Check sheet for the modelled part. Datum: model origin and axes. Units: mm. A direction names the side the tool comes from. Round coordinates to 2 decimals unless told otherwise and drop trailing zeros. Order: outer loops, then holes, each group sorted by start corner. A loop starts at its lowest first (then second) coordinate and runs counter-clockwise, first axis right, second up.
(1) Thickness scan on probe 1 along X at (y, z) = (0, -2.5); probe 2 along X at (y, z) = (0, -2.35); probe 3 along Z at (x, y) = (6, 9). Record the ranges inside material, lowest first.
(2) Tool access check on faces 1 (the flat face through (30, -30, 8)), 2 (the cylindrical face through (-8.498, 38.268, -2.26)), 3 (the cylindrical face through (37.745, 26.292, 1.958)), 4 (the cylindrical face through (33.643, -23.434, 9.86)), 5 (the conical face through (36.731, 25.586, -2.236)). Record the directions out of +Z, -Z, +X, -X, +Y, -Y that give a thin tool (end or side, any length) a straight path to the whole face; none if there is none.
(3) Sectioned sample at B-B, the plane z = 17. Count the separate pieces of the cut face and the enclosed holes in it, and give its area (3 significant figures).
(4) Sectioned sample at A-A, the plane z = 3.75. Enter the section's corners in (x, y), and give its area (3 significant figures).
(5) Mould release check, pull along X, two halves, no side actions. Record for faces 6 (the conical face through (34.102, 23.754, 19.441)), 7 (the flat face through (-36, 20, -3)), 8 (the flat face through (-30, 30, 8)): released by +X, released by -X, zero draft, split by the parting line, or undercut.
(6) Depth check by flat-ended pin: pin 1 (1 mm diameter, centred on x = -32.5, z = 8, fed in from +Y); pin 2 (1.5 mm diameter, centred on x = -15, y = -9.5, fed in from +Z); pin 3 (5 mm diameter, centred on y = 17, z = 16.5, fed in from +X). Enter the tip coordinate at first touch or a pass-through.
```python
from build123d import *
from build123d import SkipClean  # not in build123d's __all__

# Parameters (mm, degrees)
F1_DEPTH    = 20
F2_SIZE     = 4.99999
F2_2_SIZE   = 4.99999
F2_3_SIZE   = 4.99999
F2_4_SIZE   = 4.99999
F3_DEPTH    = 3
F4_SIZE     = 5
F5_R        = 41
F5_R_2      = 39.2
F6_DEPTH    = 1.5
F7_SIZE     = 5
F8_T2_ANGLE = 50
F8_T4_ANGLE = 90
F8_T6_ANGLE = 50
F8_T8_ANGLE = 90
F9_SIZE     = 2


# Not quite as in the source:
# - a fillet or chamfer that OpenCascade refuses, or shapes differently, is made with other operations: its cross-section is extruded or revolved along the edge and cut away or added
# - a fillet or chamfer is up to 0.001 mm smaller than in the source, because OpenCascade refuses the exact size


with BuildPart() as f1:
    # F0 (on Top) → F1 (new body)
    with BuildSketch(Plane.XY):
        with BuildLine():
            ThreePointArc((-37.1586192685, 17.3273487314), (-33.5852338158, 23.5166338904), (-28.9913780286, 28.9913780286))
            Line((-28.9913780286, 28.9913780286), (-32.5269119346, 32.5269119346))
            ThreePointArc((-32.5269119346, 32.5269119346), (-37.6809940373, 26.3845160721), (-41.6901582037, 19.4404400401))
            Line((-41.6901582037, 19.4404400401), (-37.1586192685, 17.3273487314))
        make_face()
    extrude(amount=F1_DEPTH)

    # F2 (size 5 in the source; OpenCascade refuses exactly that, so slightly less here)
    f2_edges = [f1.edges().sort_by_distance(p)[0] for p in [
        (-37.680994, 26.384516, 20),
    ]]
    chamfer(f2_edges, length=F2_SIZE)



with BuildPart() as f1b:
    # F0 (on Top) → F1, piece 2 (new body)
    with BuildSketch(Plane.XY):
        with BuildLine():
            ThreePointArc((28.9913780286, 28.9913780286), (33.5852338158, 23.5166338904), (37.1586192685, 17.3273487314))
            Line((37.1586192685, 17.3273487314), (41.6901582037, 19.4404400401))
            ThreePointArc((41.6901582037, 19.4404400401), (37.6809940373, 26.3845160721), (32.5269119346, 32.5269119346))
            Line((32.5269119346, 32.5269119346), (28.9913780286, 28.9913780286))
        make_face()
    extrude(amount=F1_DEPTH)

    # F2#2 (size 5 in the source; OpenCascade refuses exactly that, so slightly less here)
    f2_2_edges = [f1b.edges().sort_by_distance(p)[0] for p in [
        (37.680994, 26.384516, 20),
    ]]
    chamfer(f2_2_edges, length=F2_2_SIZE)


with BuildPart() as f1c:
    # F0 (on Top) → F1, piece 3 (new body)
    with BuildSketch(Plane.XY):
        with BuildLine():
            Line((-32.5269119346, -32.5269119346), (-28.9913780286, -28.9913780286))
            ThreePointArc((-28.9913780286, -28.9913780286), (-33.5852338158, -23.5166338904), (-37.1586192685, -17.3273487314))
            Line((-37.1586192685, -17.3273487314), (-41.6901582037, -19.4404400401))
            ThreePointArc((-41.6901582037, -19.4404400401), (-37.6809940373, -26.3845160721), (-32.5269119346, -32.5269119346))
        make_face()
    extrude(amount=F1_DEPTH)

    # F2#3 (size 5 in the source; OpenCascade refuses exactly that, so slightly less here)
    f2_3_edges = [f1c.edges().sort_by_distance(p)[0] for p in [
        (-37.680994, -26.384516, 20),
    ]]
    chamfer(f2_3_edges, length=F2_3_SIZE)


with BuildPart() as f1d:
    # F0 (on Top) → F1, piece 4 (new body)
    with BuildSketch(Plane.XY):
        with BuildLine():
            Line((41.6901582037, -19.4404400401), (37.1586192685, -17.3273487314))
            ThreePointArc((37.1586192685, -17.3273487314), (33.5852338158, -23.5166338904), (28.9913780286, -28.9913780286))
            Line((28.9913780286, -28.9913780286), (32.5269119346, -32.5269119346))
            ThreePointArc((32.5269119346, -32.5269119346), (37.6809940373, -26.3845160721), (41.6901582037, -19.4404400401))
        make_face()
    extrude(amount=F1_DEPTH)

    # F2#4 (size 5 in the source; OpenCascade refuses exactly that, so slightly less here)
    f2_4_edges = [f1d.edges().sort_by_distance(p)[0] for p in [
        (37.680994, -26.384516, 20),
    ]]
    chamfer(f2_4_edges, length=F2_4_SIZE)


with BuildPart() as f1_1:
    add(f1.part, clean=False)

    with SkipClean():  # cleaning this boolean's faces spoils the solid; the shape is the same uncleaned
        add(f1b.part)  # F3 merges F1b

    with SkipClean():  # cleaning this boolean's faces spoils the solid; the shape is the same uncleaned
        add(f1c.part)  # F3 merges F1c

    with SkipClean():  # cleaning this boolean's faces spoils the solid; the shape is the same uncleaned
        add(f1d.part)  # F3 merges F1d
    # F0 (on Top) → F3 (join)
    with BuildSketch(Plane.XY):
        with BuildLine():
            ThreePointArc((-37.1586192685, 17.3273487314), (-33.5852338158, 23.5166338904), (-28.9913780286, 28.9913780286))
            Line((-28.9913780286, 28.9913780286), (-32.5269119346, 32.5269119346))
            ThreePointArc((-32.5269119346, 32.5269119346), (-37.6809940373, 26.3845160721), (-41.6901582037, 19.4404400401))
            Line((-41.6901582037, 19.4404400401), (-37.1586192685, 17.3273487314))
        make_face()
        with BuildLine():
            Line((32.5269119346, -32.5269119346), (28.9913780286, -28.9913780286))
            ThreePointArc((28.9913780286, -28.9913780286), (0, -41), (-28.9913780286, -28.9913780286))
            Line((-28.9913780286, -28.9913780286), (-32.5269119346, -32.5269119346))
            ThreePointArc((-32.5269119346, -32.5269119346), (0, -46), (32.5269119346, -32.5269119346))
        make_face()
        with BuildLine():
            ThreePointArc((28.9913780286, 28.9913780286), (33.5852338158, 23.5166338904), (37.1586192685, 17.3273487314))
            Line((37.1586192685, 17.3273487314), (41.6901582037, 19.4404400401))
            ThreePointArc((41.6901582037, 19.4404400401), (37.6809940373, 26.3845160721), (32.5269119346, 32.5269119346))
            Line((32.5269119346, 32.5269119346), (28.9913780286, 28.9913780286))
        make_face()
        with BuildLine():
            ThreePointArc((-28.9913780286, 28.9913780286), (0, 41), (28.9913780286, 28.9913780286))
            Line((28.9913780286, 28.9913780286), (32.5269119346, 32.5269119346))
            ThreePointArc((32.5269119346, 32.5269119346), (0, 46), (-32.5269119346, 32.5269119346))
            Line((-32.5269119346, 32.5269119346), (-28.9913780286, 28.9913780286))
        make_face()
        with BuildLine():
            ThreePointArc((37.1586192685, -17.3273487314), (40.0281362919, -8.8740241715), (41, 0))
            ThreePointArc((41, 0), (40.0281362919, 8.8740241715), (37.1586192685, 17.3273487314))
            ThreePointArc((37.1586192685, 17.3273487314), (33.5852338158, 23.5166338904), (28.9913780286, 28.9913780286))
            ThreePointArc((28.9913780286, 28.9913780286), (0, 41), (-28.9913780286, 28.9913780286))
            ThreePointArc((-28.9913780286, 28.9913780286), (-33.5852338158, 23.5166338904), (-37.1586192685, 17.3273487314))
            ThreePointArc((-37.1586192685, 17.3273487314), (-41, 0), (-37.1586192685, -17.3273487314))
            ThreePointArc((-37.1586192685, -17.3273487314), (-33.5852338158, -23.5166338904), (-28.9913780286, -28.9913780286))
            ThreePointArc((-28.9913780286, -28.9913780286), (0, -41), (28.9913780286, -28.9913780286))
            ThreePointArc((28.9913780286, -28.9913780286), (33.5852338158, -23.5166338904), (37.1586192685, -17.3273487314))
        make_face()
        with BuildLine():
            Line((-32.5269119346, -32.5269119346), (-28.9913780286, -28.9913780286))
            ThreePointArc((-28.9913780286, -28.9913780286), (-33.5852338158, -23.5166338904), (-37.1586192685, -17.3273487314))
            Line((-37.1586192685, -17.3273487314), (-41.6901582037, -19.4404400401))
            ThreePointArc((-41.6901582037, -19.4404400401), (-37.6809940373, -26.3845160721), (-32.5269119346, -32.5269119346))
        make_face()
        with BuildLine():
            Line((41.6901582037, -19.4404400401), (37.1586192685, -17.3273487314))
            ThreePointArc((37.1586192685, -17.3273487314), (33.5852338158, -23.5166338904), (28.9913780286, -28.9913780286))
            Line((28.9913780286, -28.9913780286), (32.5269119346, -32.5269119346))
            ThreePointArc((32.5269119346, -32.5269119346), (37.6809940373, -26.3845160721), (41.6901582037, -19.4404400401))
        make_face()
        with BuildLine():
            ThreePointArc((37.1586192685, 17.3273487314), (40.0281362919, 8.8740241715), (41, 0))
            ThreePointArc((41, 0), (40.0281362919, -8.8740241715), (37.1586192685, -17.3273487314))
            Line((37.1586192685, -17.3273487314), (41.6901582037, -19.4404400401))
            ThreePointArc((41.6901582037, -19.4404400401), (44.9096163275, -9.9562222412), (46, 0))
            ThreePointArc((46, 0), (44.9096163275, 9.9562222412), (41.6901582037, 19.4404400401))
            Line((41.6901582037, 19.4404400401), (37.1586192685, 17.3273487314))
        make_face()
        with BuildLine():
            ThreePointArc((-37.1586192685, -17.3273487314), (-41, 0), (-37.1586192685, 17.3273487314))
            Line((-37.1586192685, 17.3273487314), (-41.6901582037, 19.4404400401))
            ThreePointArc((-41.6901582037, 19.4404400401), (-46, 0), (-41.6901582037, -19.4404400401))
            Line((-41.6901582037, -19.4404400401), (-37.1586192685, -17.3273487314))
        make_face()
    with SkipClean():  # cleaning this boolean's faces spoils the solid; the shape is the same uncleaned
        extrude(amount=-F3_DEPTH)

    # F4
    f4_edges = [f1_1.edges().sort_by_distance(p)[0] for p in [
        (-37.680994, -26.384516, 15.00001),
        (-37.680994, 26.384516, 15.00001),
        (37.680994, -26.384516, 15.00001),
        (37.680994, 26.384516, 15.00001),
    ]]
    chamfer(f4_edges, length=F4_SIZE)

    # F5 (on face) → F6 (cut)
    with BuildSketch(Plane(origin=(0, 0, -3), x_dir=(1, 0, 0), z_dir=(0, 0, -1))):
        Circle(F5_R)
        Circle(F5_R_2, mode=Mode.SUBTRACT)
    with SkipClean():  # cleaning this boolean's faces spoils the solid; the shape is the same uncleaned
        extrude(amount=-F6_DEPTH, mode=Mode.SUBTRACT)

    # F7
    f7_edges = [f1_1.edges().sort_by_distance(p)[0] for p in [
        (-37.680994, -26.384516, 10.00001),
        (37.680994, -26.384516, 10.00001),
        (37.680994, 26.384516, 10.00001),
        (-37.680994, 26.384516, 10.00001),
    ]]
    chamfer(f7_edges, length=F7_SIZE)

    # F8: chamfer of 5 on 4 edges, made by hand

    # F8_s1 → F8_t2 (revolve, cut)
    with BuildSketch(Plane(origin=(0, 0, 0), x_dir=(0, 0, 1), z_dir=(0.4226182617, 0.906307787, 0))):
        Polygon((0, -41), (-5, -46), (0, -46), align=None)
    revolve(axis=Axis((0, 0, 0), (0, 0, 1)), revolution_arc=F8_T2_ANGLE, mode=Mode.SUBTRACT)

    # F8_s3 → F8_t4 (revolve, cut)
    with BuildSketch(Plane(origin=(0, 0, 0), x_dir=(0, 0, 1), z_dir=(0.7071067812, -0.7071067812, 0))):
        Polygon((0, -41), (-5, -46), (0, -46), align=None)
    revolve(axis=Axis((0, 0, 0), (0, 0, 1)), revolution_arc=F8_T4_ANGLE, mode=Mode.SUBTRACT)

    # F8_s5 → F8_t6 (revolve, cut)
    with BuildSketch(Plane(origin=(0, 0, 0), x_dir=(0, 0, 1), z_dir=(-0.4226182617, -0.906307787, 0))):
        Polygon((0, -41), (-5, -46), (0, -46), align=None)
    revolve(axis=Axis((0, 0, 0), (0, 0, 1)), revolution_arc=F8_T6_ANGLE, mode=Mode.SUBTRACT)

    # F8_s7 → F8_t8 (revolve, cut)
    with BuildSketch(Plane(origin=(0, 0, 0), x_dir=(0, 0, 1), z_dir=(-0.7071067812, 0.7071067812, 0))):
        Polygon((0, -41), (-5, -46), (0, -46), align=None)
    revolve(axis=Axis((0, 0, 0), (0, 0, 1)), revolution_arc=F8_T8_ANGLE, mode=Mode.SUBTRACT)

    # F9
    f9_edges = [f1_1.edges().sort_by_distance(p)[0] for p in [
        (-37.680994, -26.384516, -3),
        (37.680994, -26.384516, -3),
        (37.680994, 26.384516, -3),
        (-37.680994, 26.384516, -3),
    ]]
    chamfer(f9_edges, length=F9_SIZE)


solid = f1_1.part
```
Derived:
1. probe 1: x = -43.5 to -41, -39.2 to 39.2, 41 to 43.5
1. probe 2: x = -43.35 to -41, -39.2 to 39.2, 41 to 43.35
1. probe 3: z = -3 to 0
2. face 1: +Z, -Y
2. face 2: -Z
2. face 3: +Z, -Z, +X, +Y
2. face 4: +Z
2. face 5: -Z, +X, +Y
3. separate pieces: 4
3. enclosed holes: 0
3. area: 123 mm2
4. outline: (-41.69, -19.44) arc R46 ccw to (-32.53, -32.53) - (-28.99, -28.99) arc R41 cw to (-37.16, -17.33) - close; (-41.69, 19.44) - (-37.16, 17.33) arc R41 cw to (-28.99, 28.99) - (-32.53, 32.53) arc R46 ccw to start; (28.99, -28.99) - (32.53, -32.53) arc R46 ccw to (41.69, -19.44) - (37.16, -17.33) arc R41 cw to start; (28.99, 28.99) arc R41 cw to (37.16, 17.33) - (41.69, 19.44) arc R46 ccw to (32.53, 32.53) - close
4. area: 304 mm2
5. face 6: released by +X
5. face 7: zero draft
5. face 8: undercut
6. pin 1: stops at y = 32.16
6. pin 2: stops at z = 0
6. pin 3: stops at x = 39.96
